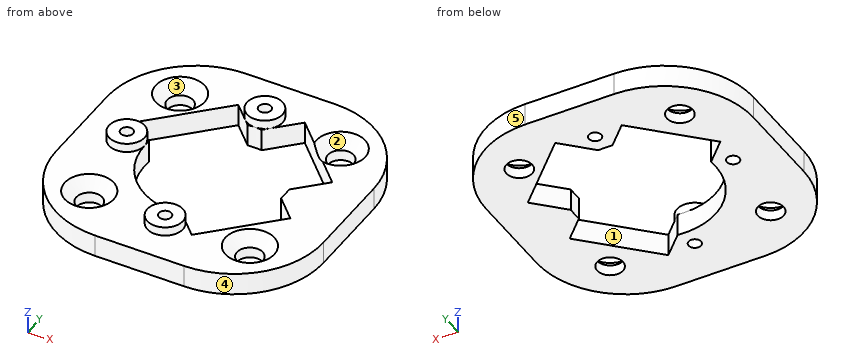
from build123d import *

# Parameters (mm, degrees)
SKETCH1_W                                      = 30
SKETCH1_H                                      = 30
BOSS_EXTRUDE1_DEPTH                            = 2.5
CUT_EXTRUDE1_DEPTH                             = 3.5
SKETCH3_W                                      = 2
SKETCH3_H                                      = 1
SKETCH4_W                                      = 2
SKETCH4_H                                      = 1
SKETCH5_W                                      = 2
SKETCH5_H                                      = 1
CSK_FOR_M2_5_FLAT_HEAD_MACHINE_SCREW1_AT_COUNT = 2
CSK_FOR_M2_5_FLAT_HEAD_MACHINE_SCREW1_AT_PITCH = 18.03122292
CSK_FOR_M2_5_FLAT_HEAD_MACHINE_SCREW_2_COUNT   = 2
CSK_FOR_M2_5_FLAT_HEAD_MACHINE_SCREW_2_PITCH   = 25.5
CSK_FOR_M2_5_FLAT_HEAD_MACHINE_SCREW_3_COUNT   = 2
CSK_FOR_M2_5_FLAT_HEAD_MACHINE_SCREW_3_PITCH   = 18.03122292
F_1_4_1_4_DIAMETER_HOLE1_D                     = 1.4
F_1_4_1_4_DIAMETER_HOLE1_DEPTH                 = 3.5
FILLET1_R                                      = 10


with BuildPart() as part:
    # Sketch1 → Boss-Extrude1 (new body)
    with BuildSketch(Plane(origin=(0, 0, 0), x_dir=(-1, 0, 0), z_dir=(0, 0, -1))):
        Rectangle(SKETCH1_W, SKETCH1_H)
    extrude(amount=-BOSS_EXTRUDE1_DEPTH)

    # Sketch2 → Cut-Extrude1 (cut, through all)
    with BuildSketch(Plane.XY.offset(2.5)):
        with BuildLine():
            Line((-3.181980515, 10.253048327), (-10.253048327, 3.181980515))
            Line((-10.253048327, 3.181980515), (-7.860000362, 0.78893255))
            ThreePointArc((-7.860000362, 0.78893255), (-5.585786438, -5.585786438), (0.78893255, -7.860000362))
            Line((0.78893255, -7.860000362), (3.181980515, -10.253048327))
            Line((3.181980515, -10.253048327), (10.253048327, -3.181980515))
            Line((10.253048327, -3.181980515), (7.860000362, -0.78893255))
            ThreePointArc((7.860000362, -0.78893255), (7.899494937, 0), (7.860000362, 0.78893255))
            Line((7.860000362, 0.78893255), (10.960155108, 3.889087297))
            Line((10.960155108, 3.889087297), (3.889087297, 10.960155108))
            Line((3.889087297, 10.960155108), (0.78893255, 7.860000362))
            ThreePointArc((0.78893255, 7.860000362), (0, 7.899494937), (-0.78893255, 7.860000362))
            Line((-0.78893255, 7.860000362), (-3.181980515, 10.253048327))
        make_face()
    extrude(amount=-CUT_EXTRUDE1_DEPTH, mode=Mode.SUBTRACT)

    # Sketch3 → Revolve1 (revolve)
    with BuildSketch(Plane.XZ):
        with Locations((-8.899494937, 3)):
            Rectangle(SKETCH3_W, SKETCH3_H)
    revolve(axis=Axis((-9.899494937, 0, 3.5), (0, 0, -1)))

    # Sketch4 → Revolve2 (revolve)
    with BuildSketch(Plane.XZ.offset(-9.899494937)):
        with Locations((1, 3)):
            Rectangle(SKETCH4_W, SKETCH4_H)
    revolve(axis=Axis((0, 9.899494937, 3.5), (0, 0, -1)))

    # Sketch5 → Revolve3 (revolve)
    with BuildSketch(Plane.XZ.offset(9.899494937)):
        with Locations((1, 3)):
            Rectangle(SKETCH5_W, SKETCH5_H)
    revolve(axis=Axis((0, -9.899494937, 3.5), (0, 0, -1)))

    # Sketch6 → CSK for M2.5 Flat Head Machine Screw1 (revolve, cut)
    with BuildSketch(Plane(origin=(9.01561146, 9.01561146, 2.5), x_dir=(0, -1, 0), z_dir=(1, 0, 0))):
        Polygon((0, 0), (0, 2.5), (1.45, 2.5), (1.45, 1.3), (2.75, 0), align=None)
    csk_for_m2_5_flat_head_machine_screw1 = revolve(axis=Axis((9.01561146, 9.01561146, 8.85), (0, 0, -1)), mode=Mode.SUBTRACT)

    # CSK for M2.5 Flat Head Machine Screw1 at: CSK for M2.5 Flat Head Machine Screw1 ×2
    with Locations(*[(-i * CSK_FOR_M2_5_FLAT_HEAD_MACHINE_SCREW1_AT_PITCH, 0, 0) for i in range(1, CSK_FOR_M2_5_FLAT_HEAD_MACHINE_SCREW1_AT_COUNT)]):
        add(csk_for_m2_5_flat_head_machine_screw1, mode=Mode.SUBTRACT)

    # CSK for M2.5 Flat Head Machine Screw 2: CSK for M2.5 Flat Head Machine Screw1 ×2
    with Locations(*[Vector(-0.707106781, -0.707106781, 0) * (i * CSK_FOR_M2_5_FLAT_HEAD_MACHINE_SCREW_2_PITCH) for i in range(1, CSK_FOR_M2_5_FLAT_HEAD_MACHINE_SCREW_2_COUNT)]):
        add(csk_for_m2_5_flat_head_machine_screw1, mode=Mode.SUBTRACT)

    # CSK for M2.5 Flat Head Machine Screw 3: CSK for M2.5 Flat Head Machine Screw1 ×2
    with Locations(*[(0, -i * CSK_FOR_M2_5_FLAT_HEAD_MACHINE_SCREW_3_PITCH, 0) for i in range(1, CSK_FOR_M2_5_FLAT_HEAD_MACHINE_SCREW_3_COUNT)]):
        add(csk_for_m2_5_flat_head_machine_screw1, mode=Mode.SUBTRACT)

    # Ø1.4 (1.4) Diameter Hole1
    with Locations(Plane(origin=(0, 0, 0), x_dir=(-1, 0, 0), z_dir=(0, 0, -1))):
        with Locations((9.899494937, 0), (0, -9.899494937), (0, 9.899494937)):
            Hole(F_1_4_1_4_DIAMETER_HOLE1_D / 2, depth=F_1_4_1_4_DIAMETER_HOLE1_DEPTH)

    # Fillet1
    fillet1_edges = [part.edges().sort_by_distance(p)[0] for p in [
        (15, -15, 1.25),
        (15, 15, 1.25),
        (-15, 15, 1.25),
        (-15, -15, 1.25),
    ]]
    fillet(fillet1_edges, radius=FILLET1_R)


solid = part.part
Geometry: final body of the model. Coordinates: model frame, mm. Face numbers are marked on the shaded views. A direction names the side the tool comes from. Coordinates: 2 decimals unless noted, no trailing zeros. Order: outer loops, then holes, each group sorted by start corner. A loop starts at its lowest first (then second) coordinate and runs counter-clockwise, first axis right, second up. Notation, with made-up numbers: M 79.5,-18.5 L 119.5,-18.5 A25 ccw 119.5,2.5 Z; hole C 64.25,22 d3. An arc over 180 degrees is marked long. One line per question, with ' | ' between items. Start each with the question number.
Item 1: Cut plane A-A, the plane y = -1.5. Return the cut outline in (x, z).
Item 2: Ray query, probe 1 along Y at (x, z) = (0, 3.25); probe 2 along Y at (x, z) = (9, 1.45); probe 3 along Y at (x, z) = (0, 2.2). Return the intervals inside material, ascending. Write a range as [from, to].
Item 3: Pin query (flat end, axial travel): pin 1 Ø2 at (x, y) = (-7.5, -2.5) entering from +Z; pin 2 Ø4.5 at (x, y) = (9.02, -9.02) entering from +Z; pin 3 Ø3.5 at (x, y) = (-9.02, 9.02) entering from +Z. Return the tip coordinate at first contact, or that it passes through.
Item 4: Set-up query: the marked faces 1 and 2. Return all of +Z, -Z, +X, -X, +Y, -Y with unobstructed straight access to the full face (end or side cutting, diameter ignored); none if empty.
Item 5: Cut plane C-C, the plane z = 2.05. Return the cut outline in (x, y), then the cut area to 3 significant figures.
Item 6: Cut plane B-B, the plane x = -2.5. Return the cut outline in (y, z), then the cut area to 3 significant figures.
Item 7: Cut plane D-D, the plane x = 5.5. Return the cut outline in (y, z).
Item 8: Draft query along Y for the marked faces 3, 4 and 5. Return one class per face: released by +Y, released by -Y, zero draft, split by the parting line, or undercut.
A:
1) outline: M -15,0 L -7.76,0 L -7.76,2.5 L -8.58,2.5 L -8.58,3.5 L -11.22,3.5 L -11.22,2.5 L -15,2.5 Z; M 8.57,0 L 15,0 L 15,2.5 L 8.57,2.5 Z
2) probe 1: y = [-11.9, -10.6], [-9.2, -7.9], [7.9, 9.2], [10.6, 11.9] | probe 2: y = [-14.17, -10.72], [-7.32, -4.44], [-1.93, 1.93], [5.85, 7.32], [10.72, 14.17] | probe 3: y = [-15, -10.6], [-9.2, -7.9], [7.9, 9.2], [10.6, 15]
3) pin 1: stops at z = 2.5 | pin 2: stops at z = 2.01 | pin 3: stops at z = 1.51
4) face 1: +Z, -Z | face 2: +Z
5) outline: M -15,-5 A10 ccw -5,-15 L 5,-15 A10 ccw 15,-5 L 15,5 A10 ccw 5,15 L -5,15 A10 ccw -15,5 Z; hole C -9.02,-9.02 d4.6; hole C -9.02,9.02 d4.6; hole C -9.9,0 d1.4; hole M -10.25,3.18 L -7.86,0.79 A7.9 ccw 0.79,-7.86 L 3.18,-10.25 L 10.25,-3.18 L 7.86,-0.79 A7.9 ccw 7.86,0.79 L 10.96,3.89 L 7.76,7.09 A2.3 ccw long 7.09,7.76 L 3.89,10.96 L 0.79,7.86 A7.9 ccw -0.79,7.86 L -3.18,10.25 Z; hole C 0,-9.9 d1.4; hole C 0,9.9 d1.4; hole C 9.02,-9.02 d4.6 | area: 472 mm2
6) outline: M -15,0 L -7.49,0 L -7.49,2.5 L -15,2.5 Z; M 9.57,0 L 15,0 L 15,2.5 L 9.57,2.5 Z | area: 32.3 mm2
7) outline: M -14.99,0 L -7.94,0 L -7.94,2.5 L -14.99,2.5 Z; M 9.35,0 L 14.99,0 L 14.99,2.5 L 9.35,2.5 Z
8) face 3: undercut | face 4: released by -Y | face 5: released by +Y
